Source: CAD feature listing. Evaluate the final solid. Frame: model axes, mm. A direction names the side the tool comes from. Coordinates: 2 decimals unless noted, no trailing zeros. Write each loop counter-clockwise with the first axis right and the second up, starting at its lowest first coordinate (ties: lowest second). Pieces come first, ordered by that corner, then holes. Notation, with made-up numbers: (-2.75, 8) - (31.25, 8) arc R6 cw to (31.25, 12) - close; hole circle Ø2 at (7.25, 45.5). An arc over 180 degrees is marked (long way). One line per item, written item: value.
Autodesk Inventor part; units mm, degrees
ref_plane "YZ Plane" through (0, 0, 0) normal (1, 0, 0) x (0, 1, 0)
ref_plane "XZ Plane" through (0, 0, 0) normal (0, 1, 0) x (-1, 0, 0)
ref_plane "XY Plane" through (0, 0, 0) normal (0, 0, 1) x (1, 0, 0)
sketch "Esboço1" plane through (0, 0, 0) normal (0, 1, 0) x (-1, 0, 0)
  line L0 (-25, 20) -> (25, 20)
  line L1 (25, 20) -> (25, -20)
  line L2 (25, -20) -> (-25, -20)
  line L3 (-25, -20) -> (-25, 20)
  line L4 (-25, 20) -> (25, -20) construction
  line L5 (25, 20) -> (-25, -20) construction
  point P0 (0, 0)
  dimension "d0" = 50
  dimension "d1" = 40
extrude "Extrusão1" add sketch "Esboço1" along normal blind 80
chamfer "Chanfro1" distance 25 angle 45 1 edges at (25, 40, 20) measured on face at (-8.3333, 26.6667, 20)
sketch "Esboço2" plane through (-25, 0, -20) normal (-1, 0, 0) x (0, 0, 1)
  line L0 (0, 80) -> (40, 80)
  line L1 (40, 80) -> (25, 80)
  line L2 (25, 80) -> (25, 40)
  line L3 (25, 40) -> (40, 40)
  line L4 (40, 40) -> (40, 80)
  point P0 (20, 0)
  dimension "d7" = 15
  dimension "d8" = 40
extrude "Extrusão2" cut sketch "Esboço2" against normal blind 80
1) Reachability of faces 1 (the flat face through (0, 80, -7)), 2 (the flat face through (-10, 40, 12)) from +Z, -Z, +X, -X, +Y, -Y: full face, straight path, thin tool, end or side. Return the list, or none.
Values found:
face 1: +Z, -Z, +X, -X, +Y
face 2: +Z, +X, -X, +Y
2) Contact query for flat-ended pins moving along their axis: P1, Ø12, axis at x = 0, y = 51, coming from the +Z side; P2, Ø4.5, axis at x = 2, z = 15.5, coming from the +Y side; P3, Ø2, axis at x = 12.5, y = 10.5, coming from the +Z side. Output: stop coordinate, or through.
Values found:
P1: z = 5
P2: y = 40
P3: z = 8.5
3) Section query B-B on y = 59. Output: boundary loops of the cut face in (x, z), then the cut area to 3 significant figures.
Values found:
outline: (-25, -20) - (25, -20) - (25, -5) - (15, 5) - (-25, 5) - close
area: 1,200 mm2
4) Section query A-A on x = 3. Output: boundary loops of the cut face in (y, z).
Values found:
outline: (0, -20) - (80, -20) - (80, 5) - (40, 5) - (40, 17) - (0, 17) - close
5) Material intervals for line 1 (Z direction, x = 10, y = 43.5); line 2 (Y direction, x = -16, z = 6.5); line 3 (X direction, y = 6, z = 5), sorted ascending.
Values found:
line 1: -20 to 5
line 2: 0 to 40
line 3: -25 to 15
6) Section query C-C on z = 0.5. Output: boundary loops of the cut face in (x, y).
Values found:
outline: (-25, 0) - (19.5, 0) - (19.5, 80) - (-25, 80) - close
7) Section query D-D on x = -8.5. Output: boundary loops of the cut face in (y, z).
Values found:
outline: (0, -20) - (80, -20) - (80, 5) - (40, 5) - (40, 20) - (0, 20) - close
